```python
from build123d import *

# Parameters (mm, degrees)
SKETCH1_W           = 18
SKETCH1_H           = 18
EXTRUDE_THIN1_DEPTH = 800
SKETCH2_W           = 20
SKETCH2_H           = 3
CUT_EXTRUDE1_DEPTH  = 10
SKETCH3_R           = 2.5
CUT_EXTRUDE2_DEPTH  = 10


with BuildPart() as part:
    # Sketch1 → Extrude-Thin1 (new body)
    with BuildSketch(Plane.XY):
        with BuildLine():
            Line((-10, 9.5), (-10, -9.5))
            ThreePointArc((-10, -9.5), (-9.853553391, -9.853553391), (-9.5, -10))
            Line((-9.5, -10), (9.5, -10))
            ThreePointArc((9.5, -10), (9.853553391, -9.853553391), (10, -9.5))
            Line((10, -9.5), (10, 9.5))
            ThreePointArc((10, 9.5), (9.853553391, 9.853553391), (9.5, 10))
            Line((9.5, 10), (-9.5, 10))
            ThreePointArc((-9.5, 10), (-9.853553391, 9.853553391), (-10, 9.5))
        make_face()
        Rectangle(SKETCH1_W, SKETCH1_H, mode=Mode.SUBTRACT)
    extrude(amount=EXTRUDE_THIN1_DEPTH)

    # Sketch2 → Cut-Extrude1 (cut)
    with BuildSketch(Plane(origin=(10, 0, 0), x_dir=(0, 0, -1), z_dir=(1, 0, 0))):
        with Locations((-150, 0)):
            Rectangle(SKETCH2_W, SKETCH2_H)
        with Locations((-400, 0)):
            Rectangle(SKETCH2_W, SKETCH2_H)
        with Locations((-650, 0)):
            Rectangle(SKETCH2_W, SKETCH2_H)
    extrude(amount=-CUT_EXTRUDE1_DEPTH, mode=Mode.SUBTRACT)

    # Sketch3 → Cut-Extrude2 (cut)
    with BuildSketch(Plane.XZ.offset(10)):
        with Locations((0, 25)):
            Circle(SKETCH3_R)
        with Locations((0, 275)):
            Circle(SKETCH3_R)
        with Locations((0, 525)):
            Circle(SKETCH3_R)
        with Locations((0, 775)):
            Circle(SKETCH3_R)
    extrude(amount=-CUT_EXTRUDE2_DEPTH, mode=Mode.SUBTRACT)


solid = part.part
```
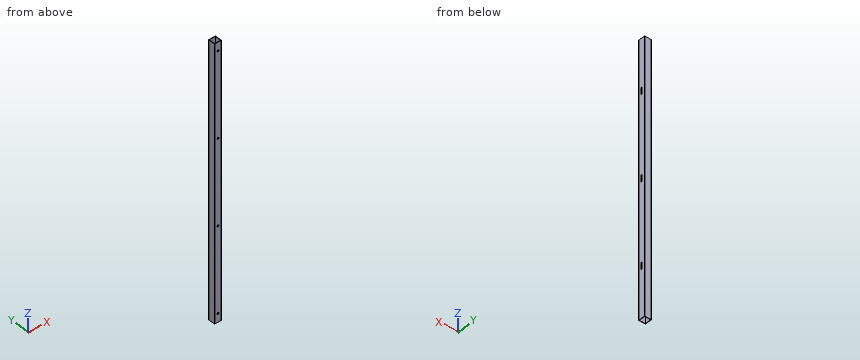
Model file for the job. Use its own axes, mm. Coordinates: 2 decimals unless noted, no trailing zeros. Write each loop counter-clockwise with the first axis right and the second up, starting at its lowest first coordinate (ties: lowest second). Pieces come first, ordered by that corner, then holes. Notation, with made-up numbers: (36.25, -24) - (51.25, -24) arc R12 cw to (51.25, -14) - close; hole circle Ø11 at (-35.75, 72). An arc over 180 degrees is marked (long way). Use a Markdown table: item, result. Add a question column.
Item 1: Band-saw the part on A-A, the plane y = -4.75. Write the cut outline in (x, z).
Item 2: Drill centre lines: line 1 along Z through (x, y) = (0, -9.4); line 2 along X through (y, z) = (2.75, 208.5). Where is each one in solid material? Low to high.
Item 3: Drop a flat-ended pin along its axis: pin 1 (3 mm diameter, centred on x = 0, z = 275, fed in from -Y). Give the stop position or say it passes through.
Item 4: Band-saw the part on B-B, the plane z = 562. Write the cut outline in (x, y).
A:
| question | item | result |
|---|---|---|
| 1 | outline | (-10, 0) - (-9, 0) - (-9, 800) - (-10, 800) - close; (9, 0) - (10, 0) - (10, 800) - (9, 800) - close |
| 2 | line 1 | z = 0 to 22.5, 27.5 to 272.5, 277.5 to 522.5, 527.5 to 772.5, 777.5 to 800 |
| 2 | line 2 | x = -10 to -9, 9 to 10 |
| 3 | pin 1 | stops at y = 9 |
| 4 | outline | (-10, -9.5) arc R0.5 ccw to (-9.5, -10) - (9.5, -10) arc R0.5 ccw to (10, -9.5) - (10, 9.5) arc R0.5 ccw to (9.5, 10) - (-9.5, 10) arc R0.5 ccw to (-10, 9.5) - close; hole (-9, -9) - (9, -9) - (9, 9) - (-9, 9) - close |
